Could you check a few things on this model? Use its own coordinates, in mm. Coordinates: 2 decimals unless noted, no trailing zeros. Order: outer loops, then holes, each group sorted by start corner. A loop starts at its lowest first (then second) coordinate and runs counter-clockwise, first axis right, second up. Notation, with made-up numbers: (80.25, 36.5) -> (100.25, 36.5) arc R28 ccw to (100.25, 73.5) -> close; hole circle Ø8 at (13, 34). An arc over 180 degrees is marked (long way). Return JSON: item names as keys, results as strings. Group by question number.
from build123d import *

# Parameters (mm, degrees)
BOSS_EXTRUDE1_DEPTH = 10
FILLET1_R           = 10
FILLET2_R           = 1
BOSS_EXTRUDE2_DEPTH = 5
CUT_EXTRUDE1_REACH  = 216.878
SKETCH3_R           = 1


with BuildPart() as part:
    # Sketch1 → Boss-Extrude1 (new body)
    with BuildSketch(Plane(origin=(0, 0, 0), x_dir=(1, 0, 0), z_dir=(0, 1, 0))):
        Polygon((-50, 11.795260846), (0, 11.795260846), (202.844423521, 66.147260317), (204.138518746, 61.317631186), (0.658262488, 6.795260846), (-50, 6.795260846), align=None)
    extrude(amount=BOSS_EXTRUDE1_DEPTH)

    # Fillet1
    fillet1_edges = [part.edges().sort_by_distance(p)[0] for p in [
        (0, 5, -11.795260846),
        (0.658262488, 5, -6.795260846),
    ]]
    fillet(fillet1_edges, radius=FILLET1_R)

    # Fillet2
    fillet2_edges = [part.edges().sort_by_distance(p)[0] for p in [
        (-25.658262488, 0, -11.795260846),
        (-25.658262488, 10, -11.795260846),
        (102.058044498, 10, -39.14163145),
        (103.034223355, 0, -34.226816884),
        (103.034223355, 10, -34.226816884),
        (0.646999434, 0, -6.880812232),
        (0.646999434, 10, -6.880812232),
        (-0.011263054, 0, -11.880812232),
        (-0.011263054, 10, -11.880812232),
        (102.058044498, 0, -39.14163145),
        (-25.329131244, 0, -6.795260846),
        (-25.329131244, 10, -6.795260846),
    ]]
    fillet(fillet2_edges, radius=FILLET2_R)

    # Sketch2 → Boss-Extrude2 (add)
    with BuildSketch(Plane.XY.offset(-6.795260846)):
        Polygon((-67.320508076, 0), (-58.660254038, -5), (-50, 0), (-50, 10), (-58.660254038, 15), (-67.320508076, 10), align=None)
        Polygon((-54.660254038, 2.690598923), (-54.660254038, 7.309401077), (-58.660254038, 9.618802154), (-62.660254038, 7.309401077), (-62.660254038, 2.690598923), (-58.660254038, 0.381197846), align=None, mode=Mode.SUBTRACT)
    extrude(amount=-BOSS_EXTRUDE2_DEPTH)

    # Sketch3 → Cut-Extrude1 (cut, up to next)
    with BuildSketch(Plane(origin=(-1.654719986, 0, -6.17549906), x_dir=(0.9659258262890681, 0, -0.2588190451025216), z_dir=(0.2588190451025216, 0, 0.9659258262890681)), mode=Mode.PRIVATE) as cut_extrude1_sk1:
        with Locations((33.711100637, 5)):
            Circle(SKETCH3_R)
    cut_extrude1_tool1 = extrude(cut_extrude1_sk1.sketch, amount=-CUT_EXTRUDE1_REACH, mode=Mode.PRIVATE) & part.part
    # Sketch3 → Cut-Extrude1 (cut, up to next)
    with BuildSketch(Plane(origin=(-1.654719986, 0, -6.17549906), x_dir=(0.9659258262890681, 0, -0.2588190451025216), z_dir=(0.2588190451025216, 0, 0.9659258262890681)), mode=Mode.PRIVATE) as cut_extrude1_sk2:
        with Locations((48.711100637, 5)):
            Circle(SKETCH3_R)
    cut_extrude1_tool2 = extrude(cut_extrude1_sk2.sketch, amount=-CUT_EXTRUDE1_REACH, mode=Mode.PRIVATE) & part.part
    # Sketch3 → Cut-Extrude1 (cut, up to next)
    with BuildSketch(Plane(origin=(-1.654719986, 0, -6.17549906), x_dir=(0.9659258262890681, 0, -0.2588190451025216), z_dir=(0.2588190451025216, 0, 0.9659258262890681)), mode=Mode.PRIVATE) as cut_extrude1_sk3:
        with Locations((63.711100637, 5)):
            Circle(SKETCH3_R)
    cut_extrude1_tool3 = extrude(cut_extrude1_sk3.sketch, amount=-CUT_EXTRUDE1_REACH, mode=Mode.PRIVATE) & part.part
    # Sketch3 → Cut-Extrude1 (cut, up to next)
    with BuildSketch(Plane(origin=(-1.654719986, 0, -6.17549906), x_dir=(0.9659258262890681, 0, -0.2588190451025216), z_dir=(0.2588190451025216, 0, 0.9659258262890681)), mode=Mode.PRIVATE) as cut_extrude1_sk4:
        with Locations((78.711100637, 5)):
            Circle(SKETCH3_R)
    cut_extrude1_tool4 = extrude(cut_extrude1_sk4.sketch, amount=-CUT_EXTRUDE1_REACH, mode=Mode.PRIVATE) & part.part
    # Sketch3 → Cut-Extrude1 (cut, up to next)
    with BuildSketch(Plane(origin=(-1.654719986, 0, -6.17549906), x_dir=(0.9659258262890681, 0, -0.2588190451025216), z_dir=(0.2588190451025216, 0, 0.9659258262890681)), mode=Mode.PRIVATE) as cut_extrude1_sk5:
        with Locations((93.711100637, 5)):
            Circle(SKETCH3_R)
    cut_extrude1_tool5 = extrude(cut_extrude1_sk5.sketch, amount=-CUT_EXTRUDE1_REACH, mode=Mode.PRIVATE) & part.part
    add(cut_extrude1_tool1.solids().sort_by_distance((30.907703, 5, -14.900574))[0], mode=Mode.SUBTRACT)
    add(cut_extrude1_tool2.solids().sort_by_distance((45.39659, 5, -18.78286))[0], mode=Mode.SUBTRACT)
    add(cut_extrude1_tool3.solids().sort_by_distance((59.885478, 5, -22.665145))[0], mode=Mode.SUBTRACT)
    add(cut_extrude1_tool4.solids().sort_by_distance((74.374365, 5, -26.547431))[0], mode=Mode.SUBTRACT)
    add(cut_extrude1_tool5.solids().sort_by_distance((88.863252, 5, -30.429717))[0], mode=Mode.SUBTRACT)


solid = part.part
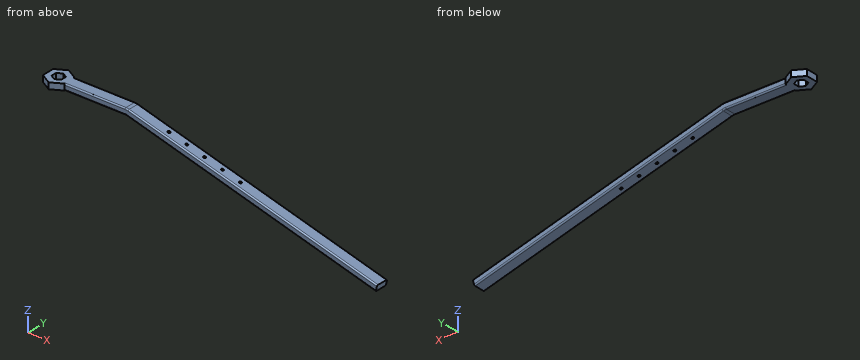
Q1. I want a section at A-A on x = -17.5. Please give me the cut outline in (y, z), and give its area (3 significant figures).
Q2. I want a section at B-B on y = -2.5. Please give me the cut outline in (x, z), and give its area (3 significant figures).
Q3. I need wall thicknesses on line 1 along Z through (x, y) = (-48, 6.75); line 2 along Y through (x, z) = (146.5, -50); line 3 along Z through (x, y) = (62.5, 1.25). Which ranges of each line are inside material? Lowest first, please. Write a range as from..to.
Q4. I'm going to push flat-ended pins straight in: pin 1 Ø4 at (x, y) = (132.5, 7.5) entering from +Z; pin 2 Ø6 at (x, y) = (-33, 6) entering from -Z; pin 3 Ø12 at (x, z) = (102.5, -30) entering from +Y. Where does each tip first touch, or does it pass through?
Response values:
{
 "1": {"outline": "(0, -10.8) arc R1 ccw to (1, -11.8) -> (9, -11.8) arc R1 ccw to (10, -10.8) -> (10, -7.8) arc R1 ccw to (9, -6.8) -> (1, -6.8) arc R1 ccw to (0, -7.8) -> close", "area": "49.1 mm²"},
 "2": {"outline": "(-62.99, -11.8) -> (-54.33, -11.8) -> (-54.33, -6.8) -> (-62.99, -6.8) -> close", "area": "43.3 mm²"},
 "3": {"line 1": "z = -11.8..-6.8", "line 2": "y = 0..10", "line 3": "z = -28.54..-23.37"},
 "4": {"pin 1": "stops at z = -41.59", "pin 2": "stops at z = -11.8", "pin 3": "stops at y = 10"}
}
